Input: part model. Units: mm. Frame: model coordinates. Face numbers are marked on the shaded views. A direction names the side the tool comes from. Coordinates: 2 decimals unless noted, no trailing zeros. Write each loop counter-clockwise with the first axis right and the second up, starting at its lowest first coordinate (ties: lowest second). Pieces come first, ordered by that corner, then holes. Notation, with made-up numbers: (22.5, 69.5) - (68.5, 69.5) arc R12 cw to (68.5, 88.5) - close; hole circle Ø5 at (-19, 38). An arc over 180 degrees is marked (long way). Put each result on its own line as item: value. Start each with the question number.
1. Access query for the marked faces 1 and 2. Directions: +Z, -Z, +X, -X, +Y, -Y. A direction counts if a zero-diameter tool reaches every point of the face in a straight line with its end or side. Return the directions, or none.
2. Cut plane B-B, the plane z = 75. Return loops of the section in (x, y).
3. Cut plane D-D, the plane y = -7. Return loops of the section in (x, z), and give its area (3 significant figures).
4. Cut plane C-C, the plane y = -3. Return loops of the section in (x, z).
5. Line query: line 1 (Y direction, x = 0, z = 34); line 2 (Z direction, x = 6.75, y = -2.5); line 3 (Z direction, x = 2.75, y = -3). Output: solid intervals per line, ascending.
6. Pin query (flat end, axial travel): pin 1 (1 mm diameter, centred on x = 1.5, z = 84.5, fed in from -Y); pin 2 (8 mm diameter, centred on y = 2.5, z = 32, fed in from -X); pin 3 (10 mm diameter, centred on x = 5.5, y = 1, fed in from +Z); pin 4 (1 mm diameter, centred on x = 1, z = 65.5, fed in from -Y). Return the tip coordinate at first contact, or that it passes through.
7. Cut plane A-A, the plane x = 2.75. Return loops of the section in (y, z), and give its area (3 significant figures).
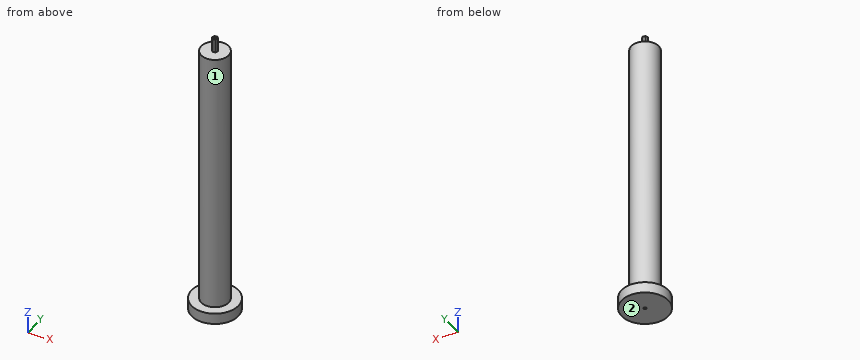
from build123d import *

# Parameters (mm, degrees)
F0_R     = 8.5
F1_DEPTH = 4
F2_R     = 5
F3_DEPTH = 100
F5_DEPTH = 5
F6_R     = 0.5
F7_DEPTH = 115.3


with BuildPart() as f1:
    # F0 (on Top) → F1 (new body)
    with BuildSketch(Plane.XY):
        Circle(F0_R)
    extrude(amount=F1_DEPTH)

    # F2 (on Top) → F3 (join)
    with BuildSketch(Plane.XY):
        Circle(F2_R)
    extrude(amount=F3_DEPTH)

    # F4 (on face) → F5 (join)
    with BuildSketch(Plane.XY.offset(100)):
        Polygon((0.674898, -0.737911), (0.976499, 0.215523), (0.301601, 0.953434), (-0.674898, 0.737911), (-0.976499, -0.215523), (-0.301601, -0.953434), align=None)
    extrude(amount=F5_DEPTH)

    # F6 (on face) → F7 (cut)
    with BuildSketch(Plane.XY.offset(105)):
        Circle(F6_R)
    extrude(amount=-F7_DEPTH, mode=Mode.SUBTRACT)


solid = f1.part
Report:
1. face 1: +Z
1. face 2: -Z, +X, -X, +Y, -Y
2. outline: circle Ø10 at (0, 0); hole circle Ø1 at (0, 0)
3. outline: (-4.82, 0) - (4.82, 0) - (4.82, 4) - (-4.82, 4) - close
3. area: 38.6 mm^2
4. outline: (-7.95, 0) - (7.95, 0) - (7.95, 4) - (4, 4) - (4, 100) - (-4, 100) - (-4, 4) - (-7.95, 4) - close
5. line 1: y = -5 to -0.5, 0.5 to 5
5. line 2: z = 0 to 4
5. line 3: z = 0 to 100
6. pin 1: stops at y = -4.9
6. pin 2: stops at x = -5
6. pin 3: stops at z = 105
6. pin 4: stops at y = -4.97
7. outline: (-8.04, 0) - (8.04, 0) - (8.04, 4) - (4.18, 4) - (4.18, 100) - (-4.18, 100) - (-4.18, 4) - (-8.04, 4) - close
7. area: 866 mm^2
